Read the model definition and answer for the solid it produces. Units are mm, in the model's axes. Round coordinates to 2 decimals unless told otherwise and drop trailing zeros. Order: outer loops, then holes, each group sorted by start corner. A loop starts at its lowest first (then second) coordinate and runs counter-clockwise, first axis right, second up.
from build123d import *

# Parameters (mm, degrees)
S01_FLAT_1_5_MM_STEEL_DISC_AND_GEARBOX_R       = 21
S01_FLAT_1_5_MM_STEEL_DISC_AND_GEARBOX_R_2     = 3.6
F_01_FLAT_1_5_MM_STEEL_DISC_AND_GEARBOX_DEPTH  = 1.5
F_02_START                                     = -0.1
S02_THREE_CARRIER_BOLTS_R                      = 1.7
F_02_THREE_CARRIER_BOLTS_DEPTH                 = 1.7
F_03_START                                     = -0.1
S03_TWO_POLOLU_FACE_SCREWS_AT_17_MM_PI_R       = 1.65
F_03_TWO_POLOLU_FACE_SCREWS_AT_17_MM_PIT_DEPTH = 1.7


with BuildPart() as part:
    # S01 - Flat 1.5 mm steel disc and gearbox pilot → 01 - Flat 1.5 mm steel disc and gearbox pilot (new body)
    with BuildSketch(Plane.XY):
        Circle(S01_FLAT_1_5_MM_STEEL_DISC_AND_GEARBOX_R)
        Circle(S01_FLAT_1_5_MM_STEEL_DISC_AND_GEARBOX_R_2, mode=Mode.SUBTRACT)
    extrude(amount=F_01_FLAT_1_5_MM_STEEL_DISC_AND_GEARBOX_DEPTH)

    # S02 - Three carrier bolts → 02 - Three carrier bolts (cut)
    with BuildSketch(Plane.XY.offset(F_02_START)):
        with Locations((14.202816622, 8.2)):
            Circle(S02_THREE_CARRIER_BOLTS_R)
        with Locations((-14.202816622, 8.2)):
            Circle(S02_THREE_CARRIER_BOLTS_R)
        with Locations((0, -16.4)):
            Circle(S02_THREE_CARRIER_BOLTS_R)
    extrude(amount=F_02_THREE_CARRIER_BOLTS_DEPTH, mode=Mode.SUBTRACT)

    # S03 - Two Pololu face screws at 17 mm pitch → 03 - Two Pololu face screws at 17 mm pitch (cut)
    with BuildSketch(Plane.XY.offset(F_03_START)):
        with Locations((0, 8.5)):
            Circle(S03_TWO_POLOLU_FACE_SCREWS_AT_17_MM_PI_R)
        with Locations((0, -8.5)):
            Circle(S03_TWO_POLOLU_FACE_SCREWS_AT_17_MM_PI_R)
    extrude(amount=F_03_TWO_POLOLU_FACE_SCREWS_AT_17_MM_PIT_DEPTH, mode=Mode.SUBTRACT)


solid = part.part
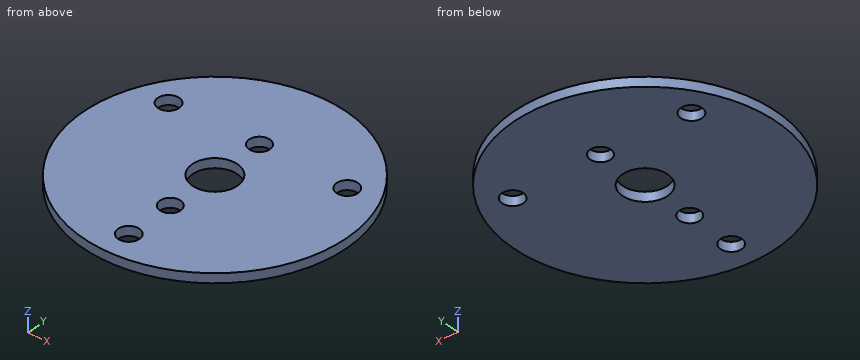
Q1. Flat-ended cylindrical pins translate along their axes: pin 1 (3 mm diameter, centred on x = 0, y = -8.5, fed in from -Z); pin 2 (12 mm diameter, centred on x = -2.5, y = -7, fed in from -Z). Find the tip coordinate at first contact, or state that the pin passes through.
Outcome:
pin 1: passes through
pin 2: stops at z = 0
Q2. A cutting plane is placed at B-B, the plane y = 0. Give the vertices of the cut face in (x, z), plus the area to 3 significant figures.
Outcome:
outline: (-21, 0) - (-3.6, 0) - (-3.6, 1.5) - (-21, 1.5) - close; (3.6, 0) - (21, 0) - (21, 1.5) - (3.6, 1.5) - close
area: 52.2 mm2
Q3. A cutting plane is placed at A-A, the plane z = 1.1. Give the vertices of the cut face in (x, y).
Outcome:
outline: circle Ø42 at (0, 0); hole circle Ø3.4 at (-14.2, 8.2); hole circle Ø7.2 at (0, 0); hole circle Ø3.4 at (0, -16.4); hole circle Ø3.3 at (0, -8.5); hole circle Ø3.3 at (0, 8.5); hole circle Ø3.4 at (14.2, 8.2)
Q4. Straight lines are drawn through the part: probe 1 along Y at (x, z) = (0, 0.45); probe 2 along Y at (x, z) = (1, 0.2); probe 3 along X at (y, z) = (8.2, 0.7). For each, find the intervals that lie inside material, in ascending order.
Outcome:
probe 1: y = -21 to -18.1, -14.7 to -10.15, -6.85 to -3.6, 3.6 to 6.85, 10.15 to 21
probe 2: y = -20.98 to -17.77, -15.03 to -9.81, -7.19 to -3.46, 3.46 to 7.19, 9.81 to 20.98
probe 3: x = -19.33 to -15.9, -12.5 to -1.62, 1.62 to 12.5, 15.9 to 19.33
Q5. A cutting plane is placed at D-D, the plane y = 9. Give the vertices of the cut face in (x, z).
Outcome:
outline: (-18.97, 0) - (-15.7, 0) - (-15.7, 1.5) - (-18.97, 1.5) - close; (-12.7, 0) - (-1.57, 0) - (-1.57, 1.5) - (-12.7, 1.5) - close; (1.57, 0) - (12.7, 0) - (12.7, 1.5) - (1.57, 1.5) - close; (15.7, 0) - (18.97, 0) - (18.97, 1.5) - (15.7, 1.5) - close
Q6. A cutting plane is placed at C-C, the plane x = 13.5. Give the vertices of the cut face in (y, z).
Outcome:
outline: (-16.09, 0) - (6.65, 0) - (6.65, 1.5) - (-16.09, 1.5) - close; (9.75, 0) - (16.09, 0) - (16.09, 1.5) - (9.75, 1.5) - close
